```python
from build123d import *

# Parameters (mm, degrees)
F0_W     = 69.85
F0_H     = 39.0903693825
F1_DEPTH = 25.4
F2_W     = 44.45
F2_H     = 25.4
F3_DEPTH = 25.4
F5_DEPTH = 25.4
F7_DEPTH = 25.4


with BuildPart() as f1:
    # F0 (on Right) → F1 (new body)
    with BuildSketch(Plane.YZ):
        with Locations((-0.1859475348, -10.3888954036)):
            Rectangle(F0_W, F0_H)
    extrude(amount=F1_DEPTH)

    # F2 (on face) → F3 (cut)
    with BuildSketch(Plane.YZ.offset(25.4)):
        with Locations((12.5140524652, -3.5437107123)):
            Rectangle(F2_W, F2_H)
    extrude(amount=-F3_DEPTH, mode=Mode.SUBTRACT)

    # F4 (on face) → F5 (cut)
    with BuildSketch(Plane.YZ.offset(25.4)):
        with BuildLine():
            Line((-9.7109475348, 9.1562892877), (-22.4109475348, 9.1562892877))
            ThreePointArc((-22.4109475348, 9.1562892877), (-13.4306914137, 5.4365454087), (-9.7109475348, -3.5437107123))
            Line((-9.7109475348, -3.5437107123), (-9.7109475348, 9.1562892877))
        make_face()
        with BuildLine():
            Line((-22.4109475348, 9.1562892877), (-35.1109475348, 9.1562892877))
            Line((-35.1109475348, 9.1562892877), (-35.1109475348, -3.5437107123))
            ThreePointArc((-35.1109475348, -3.5437107123), (-31.3912036558, 5.4365454087), (-22.4109475348, 9.1562892877))
        make_face()
        with BuildLine():
            ThreePointArc((-16.0609475348, -3.5437107123), (-22.4109475348, 2.8062892877), (-28.7609475348, -3.5437107123))
            Line((-28.7609475348, -3.5437107123), (-16.0609475348, -3.5437107123))
        make_face()
        with BuildLine():
            Line((-16.0609475348, -3.5437107123), (-28.7609475348, -3.5437107123))
            ThreePointArc((-28.7609475348, -3.5437107123), (-22.4109475348, -9.8937107123), (-16.0609475348, -3.5437107123))
        make_face()
    extrude(amount=-F5_DEPTH, mode=Mode.SUBTRACT)

    # F6 (on face) → F7 (cut)
    with BuildSketch(Plane.XY.offset(-16.2437107123)):
        with BuildLine():
            Line((12.7, 34.7390524652), (0, 34.7390524652))
            Line((0, 34.7390524652), (0, 22.0390524652))
            ThreePointArc((0, 22.0390524652), (3.7197438789, 31.0193085863), (12.7, 34.7390524652))
        make_face()
        with BuildLine():
            Line((25.4, 34.7390524652), (12.7, 34.7390524652))
            ThreePointArc((12.7, 34.7390524652), (21.6802561211, 31.0193085863), (25.4, 22.0390524652))
            Line((25.4, 22.0390524652), (25.4, 34.7390524652))
        make_face()
        with BuildLine():
            ThreePointArc((19.05, 22.0390524652), (12.7, 28.3890524652), (6.35, 22.0390524652))
            Line((6.35, 22.0390524652), (19.05, 22.0390524652))
        make_face()
        Polygon((19.05, 22.0390524652), (6.35, 22.0390524652), (6.35, 11.0405298372), (6.35, 2.9890524652), (19.05, 2.9890524652), (19.05, 11.0405298372), align=None)
        with BuildLine():
            Line((19.05, 2.9890524652), (6.35, 2.9890524652))
            ThreePointArc((6.35, 2.9890524652), (12.7, -3.3609475348), (19.05, 2.9890524652))
        make_face()
    extrude(amount=-F7_DEPTH, mode=Mode.SUBTRACT)


solid = f1.part
```
The listing builds one solid part. Answer for the finished solid, in the listing's coordinates (mm). A direction names the side the tool comes from. Give positions to 0.01 mm unless a question says otherwise; leave off trailing zeros. Order: outer loops, then holes, each group sorted by start corner. A loop starts at its lowest first (then second) coordinate and runs counter-clockwise, first axis right, second up. Notation, with made-up numbers: M 83.25,75 L 108.25,75 A28 cw 108.25,98 Z; hole C -30.75,49.25 d4. An arc over 180 degrees is marked long. Put each result on its own line as item: value. Start each with the question number.
Item 1: The part is cut by section B-B, the plane y = 17.5. Determine the outline of the cut face in (x, z), and give its area (3 significant figures).
Item 2: Which of the six approach directions +Z, -Z, +X, -X, +Y, -Y give full straight-line access (tool end or side, diameter ignored) to faces 1 (the face through (21, 12, -16.244)), 2 (the face through (13, -8, -29.934)), 3 (the face through (19.05, 12, -23))?
Item 3: The part is cut by section C-C, the plane z = -8.5. Determine the outline of the cut face in (x, y), and give its area (3 significant figures).
Item 4: The part is cut by section D-D, the plane x = 24. Determine the outline of the cut face in (y, z), and give its area (3 significant figures).
Item 5: Find the intervals of material crossed by line 1 along X through (y, z) = (7.5, -24.5); line 2 along Y through (x, z) = (16.5, -3.5); line 3 along Y through (x, z) = (4.25, -4), in increasing order.
Item 6: For a pull along X with two mould halves and no side action, classify faces 4 (the face through (12.56, -3.36, -22.99)), 5 (the face through (12.878, -16.067, -3.823)), 6 (the face through (25.4, -13, -14)) as +X half, -X half, draft (parallel to the pull), parting line (faces both ways), or undercut.
Item 7: The part is cut by section A-A, the plane x = 9.25. Determine the outline of the cut face in (y, z).
Item 8: Flat-ended cylindrical pins translate along their axes: P1, Ø1.5, axis at x = 22, y = -11.5, coming from the +Z side (3 decimals); P2, Ø1, axis at y = -22, z = -12, coming from the -X side; P3, Ø8, axis at x = 7.5, y = -5.5, coming from the +Z side; P4, Ø10, axis at x = 16, z = -7, coming from the +Y side. Find the tip coordinate at first contact, or state that the pin passes through.
Answer key:
1. outline: M 0,-29.93 L 6.35,-29.93 L 6.35,-16.24 L 0,-16.24 Z; M 19.05,-29.93 L 25.4,-29.93 L 25.4,-16.24 L 19.05,-16.24 Z
1. area: 174 mm²
2. face 1: +Z, +X, -X, +Y
2. face 2: -Z, +X, -X, +Y, -Y
2. face 3: +Z, -Z
3. outline: M 0,-35.11 L 25.4,-35.11 L 25.4,-26.38 L 0,-26.38 Z; M 0,-18.44 L 25.4,-18.44 L 25.4,-9.71 L 0,-9.71 Z
3. area: 444 mm²
4. outline: M -35.11,-29.93 L 27.84,-29.93 L 27.84,-16.24 L -9.71,-16.24 L -9.71,-3.54 A12.7 ccw -35.11,-3.54 Z; hole C -22.41,-3.54 d12.7
4. area: 1,310 mm²
5. line 1: x = 0 to 6.35, 19.05 to 25.4
5. line 2: y = -35.11 to -28.76, -16.06 to -9.71
5. line 3: y = -35.11 to -28.74, -16.08 to -9.71
6. face 4: undercut
6. face 5: draft
6. face 6: +X half
7. outline: M -35.11,-29.93 L -2.34,-29.93 L -2.34,-16.24 L -9.71,-16.24 L -9.71,-3.54 A12.7 ccw -35.11,-3.54 Z; M 27.37,-29.93 L 34.26,-29.93 L 34.26,-16.24 L 27.37,-16.24 Z; hole C -22.41,-3.54 d12.7
8. P1: stops at z = 4.075
8. P2: stops at x = 0
8. P3: stops at z = -16.24
8. P4: stops at y = -9.71
